For this review, take the finished solid that the model builds, in its own axes (mm). Face numbers are marked on the shaded views. Give positions to 0.01 mm unless a question says otherwise; leave off trailing zeros. Write each loop counter-clockwise with the first axis right and the second up, starting at its lowest first coordinate (ties: lowest second). Pieces come first, ordered by that corner, then holes. Notation, with made-up numbers: (67.5, 7) -> (99.5, 7) arc R12 ccw to (99.5, 17) -> close; hole circle Ø7 at (-3, 20.25). An arc over 180 degrees is marked (long way). Write item = value, one per line.
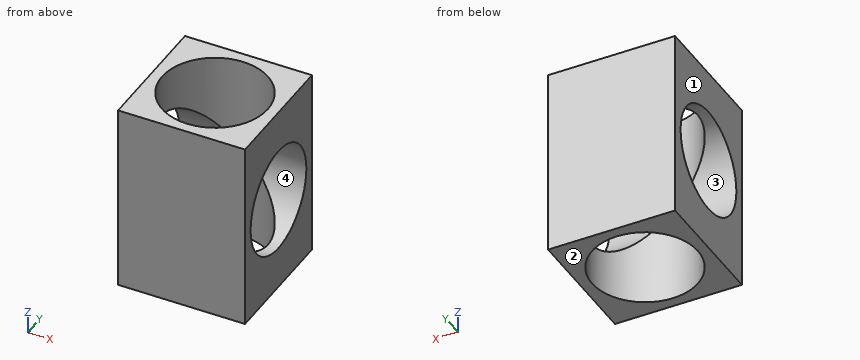
```python
from build123d import *

# Parameters (mm, degrees)
F0_W     = 60
F0_H     = 60
F0_R     = 25
F1_DEPTH = 45
F2_R     = 25
F3_DEPTH = 60.001


with BuildPart() as f1:
    # F0 (on Top) → F1 (new body, symmetric)
    with BuildSketch(Plane.XY):
        Rectangle(F0_W, F0_H)
        Circle(F0_R, mode=Mode.SUBTRACT)
    extrude(amount=F1_DEPTH, both=True)

    # F2 (on face) → F3 (cut, through all)
    with BuildSketch(Plane.YZ.offset(30)):
        Circle(F2_R)
    extrude(amount=-F3_DEPTH, mode=Mode.SUBTRACT)


solid = f1.part
```
(1) Take a section at A-A (y = 0). Write out the cut boundary in (x, z).
Answers below:
outline = (-30, -45) -> (-25, -45) -> (-25, -25) -> (-30, -25) -> close; (-30, 25) -> (-25, 25) -> (-25, 45) -> (-30, 45) -> close; (25, -45) -> (30, -45) -> (30, -25) -> (25, -25) -> close; (25, 25) -> (30, 25) -> (30, 45) -> (25, 45) -> close
(2) Take a section at B-B (z = -34.5). Write out the cut boundary in (x, y).
Answers below:
outline = (-30, -30) -> (30, -30) -> (30, 30) -> (-30, 30) -> close; hole circle Ø50 at (0, 0)
(3) The part is to be moulded in two halves that separate along Z. For the marked faces 1, 2, 3 and 4, say which applies: released by +Z, released by -Z, zero draft, split by the parting line, or undercut.
Answers below:
face_1 = zero draft
face_2 = released by -Z
face_3 = undercut
face_4 = undercut
(4) Take a section at D-D (z = 8). Write out the cut boundary in (x, y).
Answers below:
outline = (-30, -30) -> (30, -30) -> (30, -23.69) -> (8, -23.69) arc R25 cw to (-8, -23.69) -> (-30, -23.69) -> close; (-30, 23.69) -> (-8, 23.69) arc R25 cw to (8, 23.69) -> (30, 23.69) -> (30, 30) -> (-30, 30) -> close
(5) To check wall thickness, follow probe 1 along Y at (x, z) = (1, -24); probe 2 along X at (y, z) = (2, -26); probe 3 along Z at (x, y) = (24, -18). State the ranges of each line that lie inside material, in increasing order.
Answers below:
probe_1 = -30 to -24.98, 24.98 to 30
probe_2 = -30 to -24.92, 24.92 to 30
probe_3 = -45 to -17.35, 17.35 to 45
(6) Take a section at C-C (x = 5). Write out the cut boundary in (y, z), plus the area to 3 significant figures.
Answers below:
outline = (-30, -45) -> (-24.49, -45) -> (-24.49, -5) arc R25 cw to (-24.49, 5) -> (-24.49, 45) -> (-30, 45) -> close; (24.49, -45) -> (30, -45) -> (30, 45) -> (24.49, 45) -> (24.49, 5) arc R25 cw to (24.49, -5) -> close
area = 984 mm^2
